from build123d import *

# Parameters (mm, degrees)
SKETCH_2_R          = 1.5
CUT_EXTRUDE_1_DEPTH = 125.459832878


with BuildPart() as part:
    # 草图1 → 旋转1 (revolve)
    with BuildSketch(Plane.XY, mode=Mode.PRIVATE) as revolve_1_sk:
        Polygon((80.25, 0), (88, 0), (88, 2), (87, 2), (87, 1.5), (82.75, 1.5), (82.75, 2), (80.25, 2), align=None)
    revolve(revolve_1_sk.sketch.rotate(Axis((0, 155.597353718, 0), (0, -1, 0)), 90), axis=Axis((0, 155.597353718, 0), (0, -1, 0)))

    # 草图2 → 切除-拉伸1 (cut, through all)
    with BuildSketch(Plane(origin=(0, 1.5, 0), x_dir=(1, 0, 0), z_dir=(0, 1, 0))):
        with Locations(Location((0, 85.5, 0), (0, 0, 270))):
            Circle(SKETCH_2_R)
        with Locations(Location((60.457629791, 60.457629791, 0), (0, 0, 270))):
            Circle(SKETCH_2_R)
        with Locations(Location((85.5, 0, 0), (0, 0, 270))):
            Circle(SKETCH_2_R)
        with Locations(Location((60.457629791, -60.457629791, 0), (0, 0, 270))):
            Circle(SKETCH_2_R)
        with Locations(Location((0, -85.5, 0), (0, 0, 270))):
            Circle(SKETCH_2_R)
        with Locations(Location((-60.457629791, -60.457629791, 0), (0, 0, 270))):
            Circle(SKETCH_2_R)
        with Locations(Location((-85.5, 0, 0), (0, 0, 270))):
            Circle(SKETCH_2_R)
        with Locations(Location((-60.457629791, 60.457629791, 0), (0, 0, 270))):
            Circle(SKETCH_2_R)
    extrude(amount=-CUT_EXTRUDE_1_DEPTH, mode=Mode.SUBTRACT)


solid = part.part
Design review of the part built by this model. Coordinates are the model's own, in mm. A direction names the side the tool comes from. Give positions to 0.01 mm unless a question says otherwise; leave off trailing zeros. Loops run counter-clockwise (first coordinate to the right, second up) from the corner with the lowest first, then second, coordinate; pieces in that order, holes last. Notation, with made-up numbers: (-40, 24) -> (-27, 24) arc R27 ccw to (-27, 63) -> close; hole circle Ø8 at (63, 8.5). An arc over 180 degrees is marked (long way). One line per question, with ' | ' between items. Start each with the question number.
(1) Draft analysis for pull direction X (two halves, no side actions). For faces 1 (the face through (48.831, 0.986, -63.684)), 2 (the face through (85.907, 1.014, -19.077)), 3 (the face through (-20, 2, -85)), state which applies: +X half, -X half, draft (parallel to the pull), parting line (faces both ways), or undercut.
(2) We need section A-A (z = 53). State the section outline as (x, y) points.
(3) Insertion check: P1, Ø2.5, axis at x = -60.46, z = 60.46, coming from the -Y side; P2, Ø1, axis at y = 1, z = -6.5, coming from the -X side; P3, Ø1, axis at x = -64, y = 0.5, coming from the +Z side; P4, Ø1, axis at y = 0.5, z = 39, coming from the +X side. Each pin has a flat end and moves straight along its axis. Give the tip position at first contact, or say it passes through.
(4) For faces 4 (the face through (-43, 2, -68)), 5 (the face through (-86.26, 1.75, -11.33)), list the 3-axis set-ups (+Z, -Z, +X, -X, +Y, -Y) from which the entire face can be reached by the end or side of a thin tool; tool diameter is ignored.
(5) For line 1 (Z direction, x = -73, y = 1.55); line 2 (X direction, y = 1.75, z = 29.5); line 3 (X direction, y = 1.65, z = -68), list the stretches that pass through material, from the lowest coordinate up.
(6) We need section B-B (x = 10). State the section outline as (y, z) points, and give its area (3 significant figures).
The answers:
1) face 1: undercut | face 2: parting line | face 3: draft
2) outline: (-70.25, 0) -> (-60.26, 0) -> (-60.26, 2) -> (-63.55, 2) -> (-63.55, 1.5) -> (-68.99, 1.5) -> (-68.99, 2) -> (-70.25, 2) -> close; (60.26, 0) -> (70.25, 0) -> (70.25, 2) -> (68.99, 2) -> (68.99, 1.5) -> (63.55, 1.5) -> (63.55, 2) -> (60.26, 2) -> close
3) P1: passes through | P2: stops at x = -87.8 | P3: stops at z = 60.92 | P4: stops at x = 79.13
4) face 4: +Z, -Z, +X, -X, +Y | face 5: +Y
5) line 1: z = -49.14 to -47.33, -38.97 to -33.33, 33.33 to 38.97, 47.33 to 49.14 | line 2: x = -82.91 to -81.85, -77.31 to -74.63, 74.63 to 77.31, 81.85 to 82.91 | line 3: x = -55.86 to -54.27, -47.15 to -42.62, 42.62 to 47.15, 54.27 to 55.86
6) outline: (0, -87.43) -> (2, -87.43) -> (2, -86.42) -> (1.5, -86.42) -> (1.5, -82.14) -> (2, -82.14) -> (2, -79.62) -> (0, -79.62) -> close; (0, 79.62) -> (2, 79.62) -> (2, 82.14) -> (1.5, 82.14) -> (1.5, 86.42) -> (2, 86.42) -> (2, 87.43) -> (0, 87.43) -> close | area: 26.9 mm^2
